Geometry: final body of the model. Coordinates: model frame, mm. Face numbers are marked on the shaded views. A direction names the side the tool comes from. Give positions to 0.01 mm unless a question says otherwise; leave off trailing zeros. Write each loop counter-clockwise with the first axis right and the second up, starting at its lowest first coordinate (ties: lowest second). Pieces come first, ordered by that corner, then holes. Notation, with made-up numbers: M 0.25,-28.75 L 26.25,-28.75 A21 cw 26.25,-11.75 Z; hole C 13.25,89.25 d2. An arc over 180 degrees is marked long. Use one line per item in the form item = value. Start each with the question number.
Item 1: Section query D-D on x = -21. Return loops of the section in (y, z).
Item 2: Section query C-C on y = -19.75. Return loops of the section in (x, z).
Item 3: Section query A-A on x = -3. Return loops of the section in (y, z).
Item 4: Access query for the marked faces 1 and 2. Directions: +Z, -Z, +X, -X, +Y, -Y. A direction counts if a zero-diameter tool reaches every point of the face in a straight line with its end or side. Return the directions, or none.
Item 5: Section query B-B on z = -43.5. Return loops of the section in (x, y).
Item 6: Material intervals for line 1 along X through (y, z) = (-1.5, -42.5); line 2 along Z through (x, y) = (-6, -10.5); line 3 along Z through (x, y) = (-18.5, -10.5), sorted ascending. Write a range as from..to.
Item 7: Contact query for flat-ended pins moving along their axis: P1, Ø7.5, axis at y = -16, z = 31.5, coming from the -X side; P2, Ø4.5, axis at x = -34, y = -12.5, coming from the -Z side; P3, Ø4, axis at x = -43.5, y = -13, coming from the -Z side. Output: stop coordinate, or through.
Item 8: Pull-direction query (X, two-part tool) for the marked faces 3, 4 and 5; classes: released by +X, released by -X, zero draft, split by the parting line, or undercut.
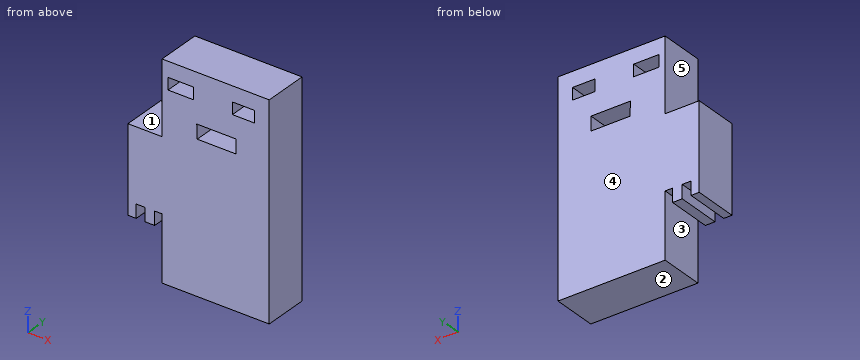
from build123d import *

# Parameters (mm, degrees)
F0_W     = 31.5706767142
F0_H     = 27.2374488413
F0_H_2   = 9.9748745561
F0_W_2   = 61.2842533737
F0_H_3   = 41.7847204953
F0_W_3   = 14.5472735167
F0_H_4   = 6.8093631417
F0_W_4   = 12.6901743934
F0_W_5   = 4.7026574612
F0_H_5   = 7.7468082309
F0_W_6   = 5.5220406502
F1_DEPTH = 25.4


with BuildPart() as f1:
    # F0 (on Front) → F1 (new body)
    with BuildSketch(Plane.XZ):
        Polygon((29.7135766596, -38.2252819836), (29.7135766596, 3.2499227673), (-31.5706767142, 3.2499227673), (-31.5706767142, -38.2252819836), (0, -38.2252819836), align=None)
        Polygon((-31.5706767142, -38.2252819836), (-31.5706767142, 3.2499227673), (-51.0702133179, 3.2499227673), (-51.0702133179, -38.2252819836), (-46.3675558567, -38.2252819836), (-41.320445016, -38.2252819836), (-35.7984043658, -38.2252819836), align=None)
        Polygon((29.7135766596, -65.4627308249), (29.7135766596, -38.2252819836), (0, -38.2252819836), (0, -65.4627308249), (2.1666167304, -65.4627308249), align=None)
        with Locations((-15.7853383571, -51.8440064043)):
            Rectangle(F0_W, F0_H)
        Polygon((29.7135766596, -75.437605381), (29.7135766596, -65.4627308249), (2.1666167304, -65.4627308249), (0, -65.4627308249), (0, -75.437605381), align=None)
        with Locations((-15.7853383571, -70.450168103)):
            Rectangle(F0_W, F0_H_2)
        with Locations((-0.9285500273, 24.142283015)):
            Rectangle(F0_W_2, F0_H_3)
        with Locations((-20.8923593163, 32.9635022208)):
            Rectangle(F0_W_3, F0_H_4, mode=Mode.SUBTRACT)
        Polygon((-11.4521086216, 9.1307349503), (-11.761624366, 17.1781629324), (-7.1188774891, 17.1781629324), (-3.7141975481, 17.1781629324), (0, 17.1781629324), (5.2617802285, 17.1781629324), (10.8330752701, 17.1781629324), (10.8330752701, 9.1307349503), (5.2617802285, 9.1307349503), (0, 9.1307349503), (-3.7141975481, 9.1307349503), (-7.1188774891, 9.1307349503), align=None, mode=Mode.SUBTRACT)
        with Locations((15.011547599, 32.9635022208)):
            Rectangle(F0_W_4, F0_H_4, mode=Mode.SUBTRACT)
        with Locations((-48.7188845873, -42.0986860991)):
            Rectangle(F0_W_5, F0_H_5)
        with Locations((-38.5594246909, -42.0986860991)):
            Rectangle(F0_W_6, F0_H_5)
    extrude(amount=F1_DEPTH)


solid = f1.part
Answer sheet:
q1.outline = M -25.4,-75.44 L 0,-75.44 L 0,29.56 L -25.4,29.56 Z; M -25.4,36.37 L 0,36.37 L 0,45.03 L -25.4,45.03 Z
q2.outline = M -51.07,-45.97 L -46.37,-45.97 L -46.37,-38.23 L -41.32,-38.23 L -41.32,-45.97 L -35.8,-45.97 L -35.8,-38.23 L -31.57,-38.23 L -31.57,-75.44 L 29.71,-75.44 L 29.71,45.03 L -31.57,45.03 L -31.57,3.25 L -51.07,3.25 Z; hole M -28.17,29.56 L -13.62,29.56 L -13.62,36.37 L -28.17,36.37 Z; hole M -11.76,17.18 L -11.45,9.13 L 10.83,9.13 L 10.83,17.18 Z; hole M 8.67,29.56 L 21.36,29.56 L 21.36,36.37 L 8.67,36.37 Z
q3.outline = M -25.4,-75.44 L 0,-75.44 L 0,9.13 L -25.4,9.13 Z; M -25.4,17.18 L 0,17.18 L 0,45.03 L -25.4,45.03 Z
q4.face_1 = +Z, -X, +Y, -Y
q4.face_2 = -Z, +X, -X, +Y, -Y
q5.outline = M -51.07,-25.4 L -46.37,-25.4 L -46.37,0 L -51.07,0 Z; M -41.32,-25.4 L -35.8,-25.4 L -35.8,0 L -41.32,0 Z; M -31.57,-25.4 L 29.71,-25.4 L 29.71,0 L -31.57,0 Z
q6.line_1 = -51.07..-46.37, -41.32..-35.8, -31.57..29.71
q6.line_2 = -75.44..9.13, 17.18..45.03
q6.line_3 = -75.44..29.56, 36.37..45.03
q7.P1 = -31.57
q7.P2 = -45.97
q7.P3 = -38.23
q8.face_3 = undercut
q8.face_4 = zero draft
q8.face_5 = released by -X
